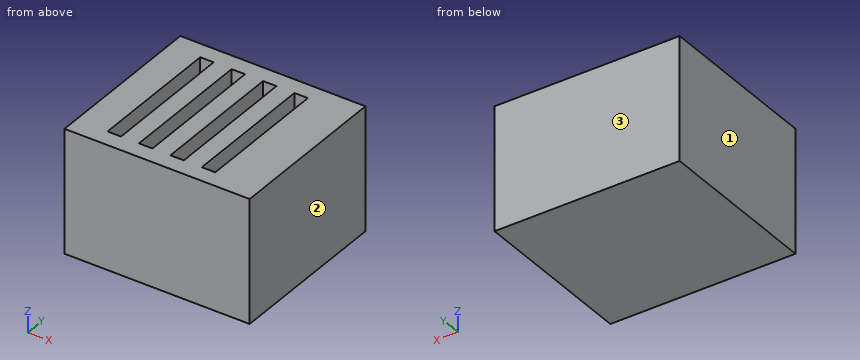
```python
from build123d import *

# Parameters (mm, degrees)
BOX004_W     = 2.4
BOX004_H     = 24
BOX004_DEPTH = 15
BOX003_W     = 2.4
BOX003_H     = 24
BOX003_DEPTH = 15
BOX001_W     = 2.4
BOX001_H     = 24
BOX001_DEPTH = 15
BOX002_W     = 2.4
BOX002_H     = 24
BOX002_DEPTH = 15
BOX_W        = 33
BOX_H        = 30
BOX_DEPTH    = 22


with BuildPart() as ranura003:
    # Box004 → Box004 (new body)
    with BuildSketch(Plane(origin=(22.4, 3, 7), x_dir=(1, 0, 0), z_dir=(0, 0, 1))):
        with Locations((1.2, 12)):
            Rectangle(BOX004_W, BOX004_H)
    extrude(amount=BOX004_DEPTH)


with BuildPart() as fusion:
    # Box003 → Box003 (new body)
    with BuildSketch(Plane(origin=(16.8, 3, 7), x_dir=(1, 0, 0), z_dir=(0, 0, 1))):
        with Locations((1.2, 12)):
            Rectangle(BOX003_W, BOX003_H)
    extrude(amount=BOX003_DEPTH)

    # Fusion: union ranura003
    add(ranura003.part)


with BuildPart() as ranura:
    # Box001 → Box001 (new body)
    with BuildSketch(Plane(origin=(5.6, 3, 7), x_dir=(1, 0, 0), z_dir=(0, 0, 1))):
        with Locations((1.2, 12)):
            Rectangle(BOX001_W, BOX001_H)
    extrude(amount=BOX001_DEPTH)


with BuildPart() as fusion002:
    # Box002 → Box002 (new body)
    with BuildSketch(Plane(origin=(11.2, 3, 7), x_dir=(1, 0, 0), z_dir=(0, 0, 1))):
        with Locations((1.2, 12)):
            Rectangle(BOX002_W, BOX002_H)
    extrude(amount=BOX002_DEPTH)

    # Fusion001: union ranura
    add(ranura.part)

    # Fusion002: union Fusion
    add(fusion.part)


with BuildPart() as cut:
    # Box → Box (new body)
    with BuildSketch(Plane.XY):
        with Locations((16.5, 15)):
            Rectangle(BOX_W, BOX_H)
    extrude(amount=BOX_DEPTH)

    # Cut: cut Fusion002
    add(fusion002.part, mode=Mode.SUBTRACT)


solid = cut.part
```
Source: CAD feature listing. Evaluate the final solid. Frame: model axes, mm. Face numbers are marked on the shaded views. Round coordinates to 2 decimals unless told otherwise and drop trailing zeros. Loops run counter-clockwise (first coordinate to the right, second up) from the corner with the lowest first, then second, coordinate; pieces in that order, holes last. Notation, with made-up numbers: (48.25, 12.25) - (53.25, 12.25) arc R25 ccw to (53.25, 29.25) - close; hole circle Ø11 at (23, 10). An arc over 180 degrees is marked (long way). Use CSV: the item, a comma, the result in double quotes.
Q1. Mould query, pull axis X, two halves, no side actions, for the marked faces 1, 2 and 3. Classes: pulls with the +X half, pulls with the -X half, needs draft (parallel to the pull), parting line crosses it, or undercut.
Reported:
face 1,"pulls with the -X half"
face 2,"pulls with the +X half"
face 3,"needs draft"
Q2. Section query B-B, the plane x = 23.5. Output: boundary loops of the cut face in (y, z), then the cut area to 3 significant figures.
Reported:
outline,"(0, 0) - (30, 0) - (30, 22) - (27, 22) - (27, 7) - (3, 7) - (3, 22) - (0, 22) - close"
area,"300 mm^2"
Q3. Pin query (flat end, axial travel): pin 1 Ø1.9 at (x, y) = (23.5, 12) entering from +Z. Return the tip coordinate at first contact, or that it passes through.
Reported:
pin 1,"z = 7"
Q4. Section query A-A, the plane z = 16.75. Output: boundary loops of the cut face in (x, y), then the cut area to 3 significant figures.
Reported:
outline,"(0, 0) - (33, 0) - (33, 30) - (0, 30) - close; hole (5.6, 3) - (8, 3) - (8, 27) - (5.6, 27) - close; hole (11.2, 3) - (13.6, 3) - (13.6, 27) - (11.2, 27) - close; hole (16.8, 3) - (19.2, 3) - (19.2, 27) - (16.8, 27) - close; hole (22.4, 3) - (24.8, 3) - (24.8, 27) - (22.4, 27) - close"
area,"760 mm^2"
Q5. Section query C-C, the plane y = 8.25. Output: boundary loops of the cut face in (x, z), then the cut area to 3 significant figures.
Reported:
outline,"(0, 0) - (33, 0) - (33, 22) - (24.8, 22) - (24.8, 7) - (22.4, 7) - (22.4, 22) - (19.2, 22) - (19.2, 7) - (16.8, 7) - (16.8, 22) - (13.6, 22) - (13.6, 7) - (11.2, 7) - (11.2, 22) - (8, 22) - (8, 7) - (5.6, 7) - (5.6, 22) - (0, 22) - close"
area,"582 mm^2"
Q6. Ray query, line 1 along X through (y, z) = (13, 7.5); line 2 along Y through (x, z) = (12, 8.75); line 3 along Z through (x, y) = (7, 25.5). Return the intervals inside material, ascending.
Reported:
line 1,"0 to 5.6, 8 to 11.2, 13.6 to 16.8, 19.2 to 22.4, 24.8 to 33"
line 2,"0 to 3, 27 to 30"
line 3,"0 to 7"
